Check sheet for the drawn part. Datum: minimum x, y, z corner. Units: mm. Give positions to 0.01 mm unless a question says otherwise; leave off trailing zeros. Write each loop counter-clockwise with the first axis right and the second up, starting at its lowest first coordinate (ties: lowest second). Pieces come first, ordered by that corner, then holes. Notation, with made-up numbers: (20.5, 73) - (74.5, 73) arc R34 ccw to (74.5, 112) - close; hole circle Ø7 at (-30.75, -8.75). An arc over 180 degrees is marked (long way). Return JSON: item names as keys, results as strings. Group by question number.
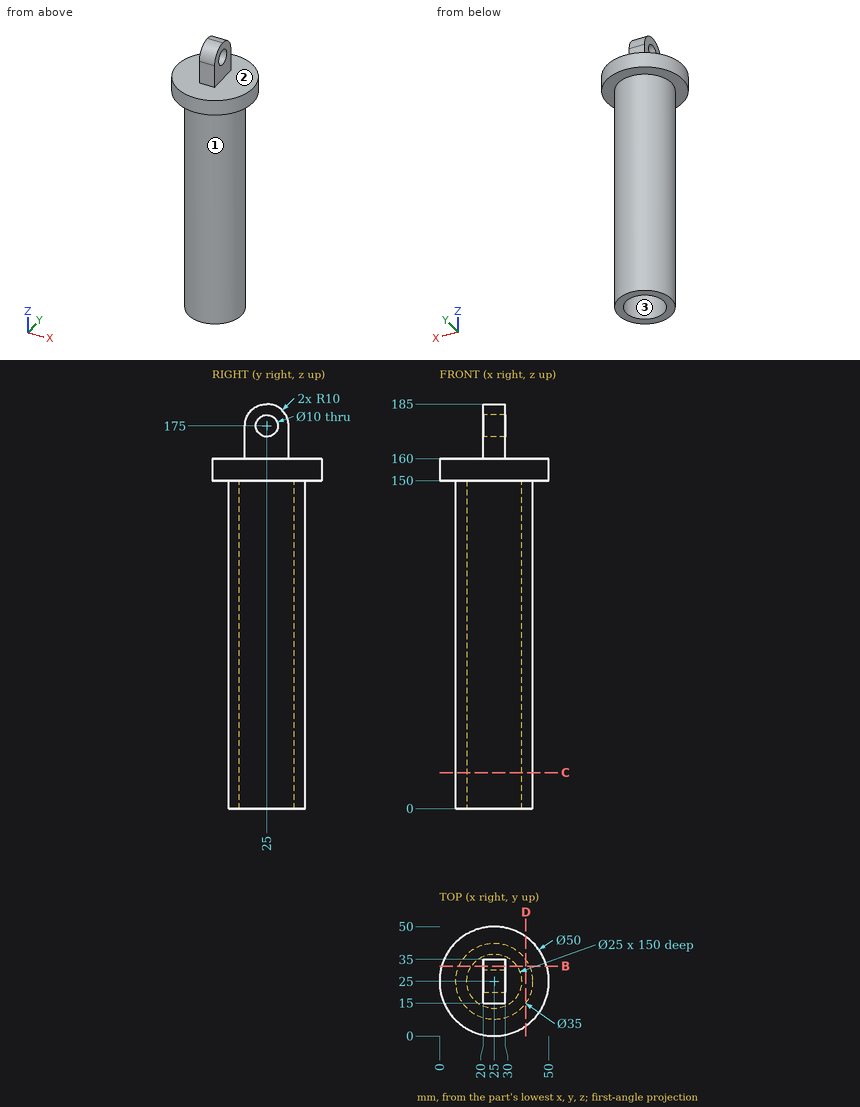
Item 1: Mould release check, pull along X, two halves, no side actions. Record for the marked faces 1, 2 and 3: +X half, -X half, draft (parallel to the pull), parting line (faces both ways), or undercut.
Item 2: Section check B-B on y = 32. Record the cut outline in (x, z), plus the area to 3 significant figures.
Item 3: Depth check by flat-ended pin: pin 1 (3 mm diameter, centred on x = 26, z = 170, fed in from +Y); pin 2 (1.5 mm diameter, centred on y = 28, z = 63, fed in from -X); pin 3 (8 mm diameter, centred on y = 13, z = 151, fed in from -X). Enter the tip coordinate at first touch or a pass-through.
Item 4: Section check C-C on z = 16.5. Record the cut outline in (x, y).
Item 5: Section check D-D on x = 39.5. Record the cut outline in (y, z).
Item 6: Material ranges on line 1 along Z through (x, y) = (27, 25); line 2 along Y through (x, z) = (25, 40); line 3 along Z through (x, y) = (18.5, 7), recorded low to high. Write a range as from..to.
Reply:
{
 "1": {"face 1": "parting line", "face 2": "draft", "face 3": "undercut"},
 "2": {"outline": "(1, 150) - (8.96, 150) - (8.96, 0) - (14.64, 0) - (14.64, 150) - (35.36, 150) - (35.36, 0) - (41.04, 0) - (41.04, 150) - (49, 150) - (49, 160) - (30, 160) - (30, 182.14) - (20, 182.14) - (20, 160) - (1, 160) - close", "area": "2,410 mm²"},
 "3": {"pin 1": "y = 35", "pin 2": "x = 7.65", "pin 3": "x = 1.31"},
 "4": {"outline": "circle Ø35 at (25, 25); hole circle Ø25 at (25, 25)"},
 "5": {"outline": "(4.63, 150) - (15.2, 150) - (15.2, 0) - (34.8, 0) - (34.8, 150) - (45.37, 150) - (45.37, 160) - (4.63, 160) - close"},
 "6": {"line 1": "150..170, 180..185", "line 2": "7.5..12.5, 37.5..42.5", "line 3": "150..160"}
}
